Input: part model. Units: mm. Frame: model coordinates. Round coordinates to 2 decimals unless told otherwise and drop trailing zeros. Loops run counter-clockwise (first coordinate to the right, second up) from the corner with the lowest first, then second, coordinate; pieces in that order, holes last.
(1) Cut plane A-A, the plane z = 1.9. Output: boundary loops of the cut face in (x, y) (3 decimals).
(2) Line query: line 1 (Y direction, x = 0, z = 1.55); line 2 (X direction, y = 6.5, z = 2.05); line 3 (X direction, y = 4.5, z = 2.6). Output: solid intervals per line, ascending.
(3) Cut plane B-B, the plane y = 1. Output: boundary loops of the cut face in (x, z), and give its area (3 significant figures).
(4) Draft query along Y for faces 1 (the face through (-7, 0, 2)), 2 (the face through (0, 8, 4)), 3 (the face through (-7.376, 6.039, 1.972)), 4 (the face through (-0.41, 3.74, 2.03)). Return one class per face: released by +Y, released by -Y, zero draft, split by the parting line, or undercut.
(5) Cut plane C-C, the plane x = 11. Output: boundary loops of the cut face in (y, z).
(6) First-contact query: pin 1 Ø2 at (x, z) = (11.5, 3.5) entering from -Y; pin 2 Ø2 at (y, z) = (3.5, 3) entering from -X; pin 3 Ø3 at (x, y) = (0, 5.6) entering from +Z; pin 4 Ø2 at (x, z) = (-3.5, 3.5) entering from +Y. Flat tips, straight axial feed; report the tip coordinate or a pass-through.
from build123d import *

# Parameters (mm, degrees)
F1_DEPTH = 4
F2_R     = 0.4
F3_R     = 1.905
F4_DEPTH = 4


with BuildPart() as f1:
    # F0 (on Top) → F1 (new body)
    with BuildSketch(Plane.XY):
        Polygon((-16, 0), (0, 0), (16, 11.203321), (0, 11.203321), align=None)
    extrude(amount=F1_DEPTH)

    # F2
    f2_edges = [f1.edges().sort_by_distance(p)[0] for p in [
        (-16, 0, 2),
        (16, 11.203321, 2),
    ]]
    fillet(f2_edges, radius=F2_R)

    # F3 (on face) → F4 (cut, through all)
    with BuildSketch(Plane.XY.offset(4)):
        with Locations((0, 5.60166)):
            Circle(F3_R)
    extrude(amount=-F4_DEPTH, mode=Mode.SUBTRACT)


solid = f1.part
Reported:
1. outline: (-14.961, 0.728) arc R0.4 ccw to (-14.731, 0) - (0, 0) - (14.961, 10.476) arc R0.4 ccw to (14.731, 11.203) - (0, 11.203) - close; hole circle Ø3.81 at (0, 5.602)
2. line 1: y = 0 to 3.7, 7.51 to 11.2
2. line 2: x = -6.72 to -1.68, 1.68 to 9.28
2. line 3: x = -9.57 to -1.55, 1.55 to 6.43
3. outline: (-14.57, 0) - (1.43, 0) - (1.43, 4) - (-14.57, 4) - close
3. area: 64.0 mm2
4. face 1: released by -Y
4. face 2: zero draft
4. face 3: released by +Y
4. face 4: undercut
5. outline: (7.7, 0) - (11.2, 0) - (11.2, 4) - (7.7, 4) - close
6. pin 1: stops at y = 7.35
6. pin 2: stops at x = -12.43
6. pin 3: passes through
6. pin 4: stops at y = 9.45
